Can you work these out from the model? Positions are in its coordinate system, mm. A direction names the side the tool comes from. Coordinates: 2 decimals unless noted, no trailing zeros. Loops run counter-clockwise (first coordinate to the right, second up) from the corner with the lowest first, then second, coordinate; pieces in that order, holes last.
```python
from build123d import *

# Parameters (mm, degrees)
SKETCH_1_R      = 2.5
EXTRUDE_1_DEPTH = 6


with BuildPart() as part:
    # 草图1 → 凸台-拉伸1 (new body)
    with BuildSketch(Plane.XY):
        with BuildLine():
            ThreePointArc((6, 29.393876913), (-30, 0), (6, -29.393876913))
            Line((6, -29.393876913), (102, -9.797958971))
            ThreePointArc((102, -9.797958971), (110, 0), (102, 9.797958971))
            Line((102, 9.797958971), (6, 29.393876913))
        make_face()
        with BuildLine():
            ThreePointArc((-13.019316478, -1.657527811), (-15.625784497, -0.715028484), (-13.11628562, 0.461575061))
            Line((-13.11628562, 0.461575061), (-1.657527811, 13.019316478))
            ThreePointArc((-1.657527811, 13.019316478), (-1.252018417, 15.499686318), (0.853539054, 14.127352485))
            ThreePointArc((0.853539054, 14.127352485), (0.752119408, 13.58515972), (0.461575061, 13.11628562))
            Line((0.461575061, 13.11628562), (13.019316478, 1.657527811))
            ThreePointArc((13.019316478, 1.657527811), (14.66954525, 2.0450413), (15.627352485, 0.646460946))
            ThreePointArc((15.627352485, 0.646460946), (14.732909957, -0.725872887), (13.11628562, -0.461575061))
            Line((13.11628562, -0.461575061), (1.657527811, -13.019316478))
            ThreePointArc((1.657527811, -13.019316478), (2.018794779, -13.521795014), (2.146460946, -14.127352485))
            ThreePointArc((2.146460946, -14.127352485), (0.104268181, -15.525932839), (-0.461575061, -13.11628562))
            Line((-0.461575061, -13.11628562), (-13.019316478, -1.657527811))
        make_face(mode=Mode.SUBTRACT)
        with Locations((100, 0)):
            Circle(SKETCH_1_R, mode=Mode.SUBTRACT)
    extrude(amount=EXTRUDE_1_DEPTH)


solid = part.part
```
Item 1: Suppose I cut it at A-A, the plane z = 4.25. Please give me the cut outline in (x, y).
Results are:
outline: (6, -29.39) - (102, -9.8) arc R10 ccw to (102, 9.8) - (6, 29.39) arc R30 ccw (long way) to start; hole (-13.12, 0.46) arc R1.5 ccw (long way) to (-13.02, -1.66) - (-0.46, -13.12) arc R1.5 ccw (long way) to (1.66, -13.02) - (13.12, -0.46) arc R1.5 ccw (long way) to (13.02, 1.66) - (0.46, 13.12) arc R1.5 ccw (long way) to (-1.66, 13.02) - close; hole circle Ø5 at (100, 0)
Item 2: We'd pull the mould along Y, two halves only. Please class faces 1 (the face through (-6.65, -7.47, 2.96)), 2 (the face through (23, 0, 0)), 3 (the face through (54.67, 19.46, 2.96)), 4 (the face through (53.328, -19.733, 2.958)): +Y half, -Y half, draft (parallel to the pull), parting line (faces both ways), or undercut.
Results are:
face 1: undercut
face 2: draft
face 3: +Y half
face 4: -Y half
Item 3: I need wall thicknesses on line 1 along X through (y, z) = (1, 1.2); line 2 along Y through (x, z) = (1, 0.8); line 3 along X through (y, z) = (-8, 2.35). Which ranges of each line are inside material? Lowest first, please.
Results are:
line 1: x = -29.98 to -12.62, 15.59 to 97.71, 102.29 to 109.95
line 2: y = -29.98 to -15.59, 12.62 to 29.98
line 3: x = -28.91 to -6.07, 6.24 to 106
Item 4: Suppose I cut it at D-D, the plane x = 65.5. Please give me the cut outline in (y, z).
Results are:
outline: (-17.25, 0) - (17.25, 0) - (17.25, 6) - (-17.25, 6) - close
Item 5: Suppose I cut it at B-B, the plane x = 100. Please give me the cut outline in (y, z).
Results are:
outline: (-10.21, 0) - (-2.5, 0) - (-2.5, 6) - (-10.21, 6) - close; (2.5, 0) - (10.21, 0) - (10.21, 6) - (2.5, 6) - close
Item 6: Suppose I cut it at C-C, the plane y = -17.5. Please give me the cut outline in (x, z).
Results are:
outline: (-24.37, 0) - (64.27, 0) - (64.27, 6) - (-24.37, 6) - close
Item 7: I'm going to push flat-ended pins straight in: P1, Ø1.5, axis at y = -7, z = 2, coming from the +X side; P2, Ø2, axis at y = -13, z = 1, coming from the -X side. Where does each tip first touch, or does it pass through?
Results are:
P1: stops at x = 107.81
P2: stops at x = -27.5
Item 8: On a 3-axis mill with a long thin cutter (end or side, diameter ignored), from which of +Z, -Z, +X, -X, +Y, -Y can I reach the whole of each face in a straight line? I mean faces 5 (the face through (23, 0, 6)), 6 (the face through (-7.47, 6.65, 2.96)). Say none if no direction works.
Results are:
face 5: +Z, +X, -X, +Y, -Y
face 6: +Z, -Z
